Verification items for the finished model (mm, model axes). A direction names the side the tool comes from. Round coordinates to 2 decimals unless told otherwise and drop trailing zeros. Answer as a JSON object with one key per item and string values. Group by question number.
```python
from build123d import *

# Parameters (mm, degrees)
SKETCH1_W                       = 538
SKETCH1_H                       = 65
EXTRUDE1_DEPTH                  = 9.525
M6X1_0_TAPPED_HOLE1_D           = 5
M6X1_0_TAPPED_HOLE1_DEPTH       = 16.9926
M6X1_0_TAPPED_HOLE1_CBORE_D     = 6
M6X1_0_TAPPED_HOLE1_CBORE_DEPTH = 11.9888
M6X1_0_TAPPED_HOLE1_TIP         = 1.502151548
CBORE_FOR_M6_SHCS1_D            = 6.6
CBORE_FOR_M6_SHCS1_CBORE_D      = 11
CBORE_FOR_M6_SHCS1_CBORE_DEPTH  = 6.762
CHAMFER1_SIZE                   = 1.27


with BuildPart() as part:
    # Sketch1 → Extrude1 (new body)
    with BuildSketch(Plane(origin=(0, 0, 0), x_dir=(1, 0, 0), z_dir=(0, 1, 0))):
        Rectangle(SKETCH1_W, SKETCH1_H)
    extrude(amount=-EXTRUDE1_DEPTH)

    # M6x1.0 Tapped Hole1
    with Locations(Plane(origin=(0, 0, 0), x_dir=(-1, 0, 0), z_dir=(0, 1, 0))):
        with Locations((178.004380433, 12.6), (178.004380433, -12.6), (77.928380433, 12.6), (77.928380433, -12.6), (-22.147619567, 12.6), (-22.147619567, -12.6), (-122.223619567, 12.6), (-122.223619567, -12.6), (-222.299619567, 12.6), (-222.299619567, -12.6)):
            CounterBoreHole(M6X1_0_TAPPED_HOLE1_D / 2, M6X1_0_TAPPED_HOLE1_CBORE_D / 2, M6X1_0_TAPPED_HOLE1_CBORE_DEPTH, depth=M6X1_0_TAPPED_HOLE1_DEPTH)
            with Locations((0, 0, -(M6X1_0_TAPPED_HOLE1_DEPTH + M6X1_0_TAPPED_HOLE1_TIP / 2))):  # 118° drill point
                Cone(0, M6X1_0_TAPPED_HOLE1_D / 2, M6X1_0_TAPPED_HOLE1_TIP, mode=Mode.SUBTRACT)

    # CBORE for M6 SHCS1 (through all)
    with Locations(Plane(origin=(0, 0, 0), x_dir=(-1, 0, 0), z_dir=(0, 1, 0))):
        with Locations((249.493618693, 12.5), (224.493618693, 12.5), (224.493618693, -12.5), (249.493618693, -12.5), (-243.6, 12.5), (-200.42, 12.5), (-243.6, -12.5), (-200.42, -12.5)):
            CounterBoreHole(CBORE_FOR_M6_SHCS1_D / 2, CBORE_FOR_M6_SHCS1_CBORE_D / 2, CBORE_FOR_M6_SHCS1_CBORE_DEPTH)

    # Chamfer1
    chamfer1_edges = [part.edges().sort_by_distance(p)[0] for p in [
        (269, -9.525, 0),
        (0, -9.525, -32.5),
        (-269, -9.525, 0),
        (0, 0, -32.5),
        (269, 0, 0),
        (0, 0, 32.5),
        (-269, 0, 0),
        (0, -9.525, 32.5),
        (-269, -4.7625, -32.5),
        (269, -4.7625, -32.5),
        (269, -4.7625, 32.5),
        (-269, -4.7625, 32.5),
    ]]
    chamfer(chamfer1_edges, length=CHAMFER1_SIZE)


solid = part.part
```
Q1. Thickness scan on line 1 (Z direction, x = 243.6, y = -4.25); line 2 (X direction, y = -6.25, z = 9.5); line 3 (Z direction, x = -180, y = -2.25). Record the ranges inside material, lowest first. Write a range as from..to.
Q2. Tool access check on faces 3 (the face through (-252, -6.762, 10)), 4 (the face through (-4, 0, 0)). Record the directions out of +Z, -Z, +X, -X, +Y, -Y that give a thin tool (end or side, any length) a straight path to the whole face; none if there is none.
Q3. Release check for a two-part mould opening along Z. For faces 1 (the face through (-229.574, -3.334, 10.393)), 2 (the face through (-4, -9.525, 0)) record: released by +Z, released by -Z, zero draft, split by the parting line, or undercut.
Q4. Gauge pin test, flat ends, axial feed: pin 1 Ø12 at (x, z) = (-223, 13) entering from +Y; pin 2 Ø5.5 at (x, z) = (-249.5, 14) entering from +Y. Record the tip position at first contact, or that the pin passes through.
Q5. Cross-section at A-A, the plane y = -3.5. Give the number of separate pieces and of enclosed holes in the cut face, then the cut area to 3 significant figures.
Conclusion:
{
 "1": {"line 1": "-32.5..-18, -7..7, 18..32.5", "line 2": "-269..-254.1, -244.88..-229.1, -219.88..195.81, 205.03..238.99, 248.21..269", "line 3": "-32.5..-14.84, -10.36..10.36, 14.84..32.5"},
 "2": {"face 3": "+Y", "face 4": "+Z, -Z, +X, -X, +Y"},
 "3": {"face 1": "undercut", "face 2": "zero draft"},
 "4": {"pin 1": "y = 0", "pin 2": "y = -6.76"},
 "5": {"separate pieces": "1", "enclosed holes": "18", "area": "33,900 mm2"}
}
